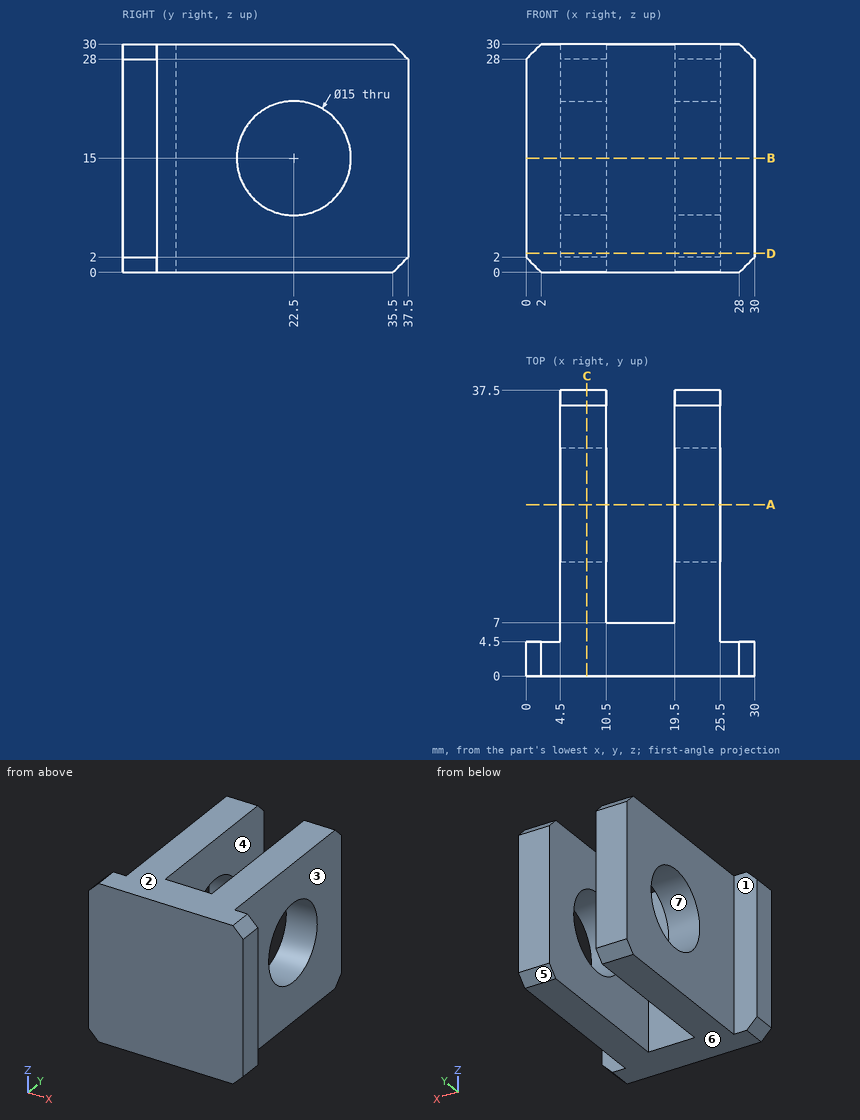
Verification items for this drawing (mm, ordinates from the low corner). A direction names the side the tool comes from. Give positions to 0.01 mm unless a question says otherwise; leave off trailing zeros. Write each loop counter-clockwise with the first axis right and the second up, starting at its lowest first coordinate (ties: lowest second). Pieces come first, ordered by that corner, then holes.
1) Section check C-C, the plane x = 8. Record the boundary of the cut face in (y, z).
2) Section check D-D, the plane z = 2.5. Record the boundary of the cut face in (x, y).
3) Release check for a two-part mould opening along Y. For the marked faces 5, 6 and 7 record: pulls with the +Y half, pulls with the -Y half, needs draft (parallel to the pull), parting line crosses it, or undercut.
4) Gauge pin test, flat ends, axial feed: pin 1 (5 mm diameter, centred on y = 25, z = 9, fed in from +X); pin 2 (2 mm diameter, centred on y = 21, z = 9.5, fed in from +X); pin 3 (9 mm diameter, centred on y = 25.5, z = 11.5, fed in from -X); pin 4 (10 mm diameter, centred on x = 14.5, z = 22, fed in from +Y). Record the tip position at first contact, or that the pin passes through.
5) Section check A-A, the plane y = 22.5. Record the boundary of the cut face in (x, z).
6) Material ranges on L1, parallel to X at y = 12.5, z = 6.75; L2, parallel to Y at x = 5.85, z = 15; L3, parallel to Z at x = 20.5, y = 16.5, recorded low to high.
7) Section check B-B, the plane z = 15. Record the boundary of the cut face in (x, y), and give its area (4 significant figures).
8) Access from +Z, -Z, +X, -X, +Y, -Y to the whole of each face (thin tool, end or side, straight path). Record for the marked faces 1, 2, 3 and 4.
Computed:
1. outline: (0, 0) - (35.5, 0) - (37.5, 2) - (37.5, 28) - (35.5, 30) - (0, 30) - close; hole circle Ø15 at (22.5, 15)
2. outline: (0, 0) - (30, 0) - (30, 4.5) - (25.5, 4.5) - (25.5, 37.5) - (19.5, 37.5) - (19.5, 7) - (10.5, 7) - (10.5, 37.5) - (4.5, 37.5) - (4.5, 4.5) - (0, 4.5) - close
3. face 5: pulls with the +Y half
3. face 6: needs draft
3. face 7: undercut
4. pin 1: stops at x = 25.5
4. pin 2: passes through
4. pin 3: stops at x = 4.5
4. pin 4: stops at y = 37.5
5. outline: (4.5, 0) - (10.5, 0) - (10.5, 7.5) - (4.5, 7.5) - close; (4.5, 22.5) - (10.5, 22.5) - (10.5, 30) - (4.5, 30) - close; (19.5, 0) - (25.5, 0) - (25.5, 7.5) - (19.5, 7.5) - close; (19.5, 22.5) - (25.5, 22.5) - (25.5, 30) - (19.5, 30) - close
6. L1: x = 4.5 to 10.5, 19.5 to 25.5
6. L2: y = 0 to 15, 30 to 37.5
6. L3: z = 0 to 10.5, 19.5 to 30
7. outline: (0, 0) - (30, 0) - (30, 4.5) - (25.5, 4.5) - (25.5, 15) - (19.5, 15) - (19.5, 7) - (10.5, 7) - (10.5, 15) - (4.5, 15) - (4.5, 4.5) - (0, 4.5) - close; (4.5, 30) - (10.5, 30) - (10.5, 37.5) - (4.5, 37.5) - close; (19.5, 30) - (25.5, 30) - (25.5, 37.5) - (19.5, 37.5) - close
7. area: 373.5 mm2
8. face 1: +Z, -Z, -X, +Y
8. face 2: +Z, +X, -X, +Y, -Y
8. face 3: +Z, -Z, +X, +Y
8. face 4: +Z, -Z, +Y
